Can you work these out from the model? Positions are in its coordinate system, mm. A direction names the side the tool comes from. Round coordinates to 2 decimals unless told otherwise and drop trailing zeros. Write each loop counter-clockwise with the first axis right and the second up, starting at its lowest first coordinate (ties: lowest second). Pieces come first, ordered by that corner, then holes. Notation, with made-up numbers: M 26,84 L 85,84 A12 ccw 85,105 Z; hole C -8.5,-30.75 d6. An arc over 180 degrees is marked long. Answer as a JSON object with one key per item and string values. Group by question number.
1) On a 3-axis mill with a long thin cutter (end or side, diameter ignored), from which of +Z, -Z, +X, -X, +Y, -Y can I reach the whole of each face in a straight line? I mean faces 1 (the cylindrical face through (-28.48, 1.92, 5.1)), 2 (the flat face through (-24.42, 5.32, 11.51)), 3 (the cylindrical face through (3.74, 8.56, 14.19)), 4 (the flat face through (0, 6, 4)). Say none if no direction works.
2) Suppose I cut it at B-B, the plane y = 3. Write out the boundary of the cut face in (x, z) (3 decimals), and give its area (3 significant figures).
3) Suppose I cut it at C-C, the plane x = -9. Write out the boundary of the cut face in (y, z), and give its area (3 significant figures).
4) If we mould it in two halves opening along X, with no side actions, what happens to faces 5 (the cylindrical face through (24.95, 4.96, 5.42)), 6 (the flat face through (-30, 3, 6)), 7 (the flat face through (1.747, 23.721, 22.947))? For each: +X half, -X half, draft (parallel to the pull), parting line (faces both ways), or undercut.
5) Please list where these lines run through material, in increasing order: L1, parallel to Y at x = 2.5, z = 8.5; L2, parallel to Y at x = 26, z = 3; L3, parallel to X at y = 15.5, z = 20. Write a range as [from, to].
6) I'm going to push flat-ended pins straight in: pin 1 Ø9 at (x, z) = (24.58, 4.23) entering from +Y; pin 2 Ø6.5 at (x, z) = (-25, 3) entering from -Y; pin 3 Ø4 at (x, y) = (4, 20) entering from +Z; pin 4 Ø3 at (x, y) = (22, 8.5) entering from +Z. Where does each tip first touch, or does it pass through?
7) Suppose I cut it at A-A, the plane x = -2.5. Write out the boundary of the cut face in (y, z), and give its area (3 significant figures).
from build123d import *

# Parameters (mm, degrees)
BOSS_EXTRUDE1_DEPTH = 30
SKETCH3_R           = 1.1
SKETCH3_R_2         = 14.25
CUT_EXTRUDE1_DEPTH  = 53.348964562
FILLET2_R           = 4
CUT_EXTRUDE2_DEPTH  = 53.378356962
SKETCH5_R           = 1.25
CUT_EXTRUDE3_DEPTH  = 50.551443345
SKETCH6_R           = 4
CUT_EXTRUDE4_DEPTH  = 3.9
CUT_EXTRUDE5_START  = -5.191520443
CUT_EXTRUDE5_DEPTH  = 0.58471683


# Read off the part's stored shape, not the designer's step: Cut-Extrude5
with BuildPart() as part:
    # Sketch1 → Boss-Extrude1 (new, symmetric)
    with BuildSketch(Plane(origin=(0, 0, 0), x_dir=(0, 0, -1), z_dir=(1, 0, 0))):
        Polygon((0, 0), (-10, 0), (-30.501566051, 29.279270691), (-28.044109918, 31), (-10.538921463, 6), (0, 6), align=None)
    extrude(amount=BOSS_EXTRUDE1_DEPTH, both=True)

    # Sketch3 → Cut-Extrude1 (cut, through all)
    with BuildSketch(Plane(origin=(0, -4.698463104, 6.710100717), x_dir=(1, 0, 0), z_dir=(0, -0.5735764363510448, 0.8191520442889928))):
        with Locations(Location((3, 38.337424669, 0), (0, 0, 270))):
            Circle(SKETCH3_R)
        with Locations(Location((27, 38.337424669, 0), (0, 0, 270))):
            Circle(SKETCH3_R)
        with Locations(Location((27, 14.337424669, 0), (0, 0, 270))):
            Circle(SKETCH3_R)
        with Locations(Location((3, 14.337424669, 0), (0, 0, 270))):
            Circle(SKETCH3_R)
        with Locations(Location((15, 26.337424669, 0), (0, 0, 270))):
            Circle(SKETCH3_R_2)
    extrude(amount=-CUT_EXTRUDE1_DEPTH, mode=Mode.SUBTRACT)

    # Fillet2
    fillet2_edges = [part.edges().sort_by_distance(p)[0] for p in [
        (0, 6, 10.538921463),
    ]]
    fillet(fillet2_edges, radius=FILLET2_R)

    # Sketch4 → Cut-Extrude2 (cut, through all)
    with BuildSketch(Plane(origin=(0, -2.977733795, 4.252644584), x_dir=(-1, 0, 0), z_dir=(0, 0.5735764363510438, -0.8191520442889935))):
        with BuildLine():
            Line((4, 41.479154), (4, 25.942790865))
            ThreePointArc((4, 25.942790865), (8.399400202, 15.347179418), (18.999990368, 10.959789281))
            Line((18.999990368, 10.959789281), (30, 10.959789281))
            Line((30, 10.959789281), (30, 41.479154))
            Line((30, 41.479154), (4, 41.479154))
        make_face()
    extrude(amount=-CUT_EXTRUDE2_DEPTH, mode=Mode.SUBTRACT)

    # Sketch5 → Cut-Extrude3 (cut, through all)
    with BuildSketch(Plane(origin=(0, 6, 0), x_dir=(1, 0, 0), z_dir=(0, 1, 0))):
        with Locations(Location((-24.575, -4.22832663, 0), (0, 0, 270))):
            Circle(SKETCH5_R)
        with Locations(Location((24.575, -4.22832663, 0), (0, 0, 270))):
            Circle(SKETCH5_R)
    extrude(amount=-CUT_EXTRUDE3_DEPTH, mode=Mode.SUBTRACT)

    # Sketch6 → Cut-Extrude4 (cut)
    with BuildSketch(Plane.XZ):
        with Locations(Location((-24.575, 4.22832663, 0), (0, 0, 270))):
            Circle(SKETCH6_R)
        with Locations(Location((24.575, 4.22832663, 0), (0, 0, 270))):
            Circle(SKETCH6_R)
    extrude(amount=-CUT_EXTRUDE4_DEPTH, mode=Mode.SUBTRACT)

    # Cut-Extrude5 outline → Cut-Extrude5 (cut)
    with BuildSketch(Plane(origin=(0, 0, 0), x_dir=(1, 0, 0), z_dir=(0, 0.5735764363510437, -0.8191520442889935)).offset(CUT_EXTRUDE5_START)):
        with BuildLine():
            ThreePointArc((-10, -13.959782058), (-14.256579589, -11.729537907), (-18.999990368, -10.959789281))
            Line((-18.999990368, -10.959789281), (-31, -10.959789281))
            Line((-31, -10.959789281), (-31, -15))
            Line((-31, -15), (-10, -15))
            Line((-10, -15), (-10, -13.959782058))
        make_face()
    extrude(amount=CUT_EXTRUDE5_DEPTH, mode=Mode.SUBTRACT)


solid = part.part
Results:
{
 "1": {"face 1": "-Y", "face 2": "+Z, -X, +Y", "face 3": "none", "face 4": "-Z, +X, -X, +Y"},
 "2": {"outline": "M -30,0 L 30,0 L 30,12.101 L -30,12.101 Z; hole C -24.575,4.228 d8; hole C 24.575,4.228 d8", "area": "626 mm^2"},
 "3": {"outline": "M 0,0 L 6,0 L 6,8.46 A4 cw 7.71,11.73 L 9.13,12.73 L 7.41,15.19 L 0,10 Z", "area": "81.6 mm^2"},
 "4": {"face 5": "undercut", "face 6": "-X half", "face 7": "draft"},
 "5": {"L1": "[0, 6]", "L2": "[3.9, 6]", "L3": "[-4.11, 0.92], [29.08, 30]"},
 "6": {"pin 1": "y = 6.01", "pin 2": "y = 0", "pin 3": "through", "pin 4": "z = 14.82"},
 "7": {"outline": "M 0,0 L 6,0 L 6,8.46 A4 cw 7.71,11.73 L 31,28.04 L 29.28,30.5 L 0,10 Z", "area": "162 mm^2"}
}
